Input: part model. Units: mm. Frame: model coordinates. A direction names the side the tool comes from. Coordinates: 2 decimals unless noted, no trailing zeros. Order: outer loops, then holes, each group sorted by start corner. A loop starts at its lowest first (then second) coordinate and runs counter-clockwise, first axis right, second up. Notation, with made-up numbers: M 6,19 L 29,19 A12 ccw 29,34 Z; hole C 16.5,17 d2. An arc over 180 degrees is marked long. Answer in a Markdown table with one row per item.
Autodesk Fusion 360 part; units mm, degrees
sketch "Sketch1" plane through (0, 0, 0) normal (0, 0, 1) x (1, 0, 0)
  line L0 (0, 0) -> (125, 0)
  line L1 (125, 0) -> (125, 65)
  line L2 (125, 65) -> (0, 65)
  line L3 (0, 65) -> (0, 0)
extrude "Extrude1" add sketch "Sketch1" along normal blind 30
sketch "Sketch2" plane through (0, 0, 0) normal (-1, 0, 0) x (0, -1, 0)
  line L0 (-65, 0) -> (0, 0)
  line L1 (0, 0) -> (0, 30)
  line L2 (0, 30) -> (-65, 30)
  line L3 (-65, 30) -> (-65, 0)
  line L4 (-20, 0) -> (-20, 15)
  line L5 (-20, 15) -> (-25, 15)
  line L6 (-25, 15) -> (-25, 25)
  line L7 (-25, 25) -> (-40, 25)
  line L8 (-40, 25) -> (-40, 15)
  line L9 (-40, 15) -> (-45, 15)
  line L10 (-45, 15) -> (-45, 0)
  line L11 (-45, 0) -> (-20, 0)
  dimension "d18" = 15
  dimension "d19" = 15
extrude "Extrude2" cut sketch "Sketch2" against normal blind 125 contours L0 L4 L5 L6 L7 L8 L9 L10 L11
extrude "Extrude3" cut 1 faces at (41.6667, 0, 10) along direction (0, 1, 0) blind 5
extrude "Extrude4" cut 1 faces at (83.3333, 65, 10) along direction (0, -1, 0) blind 5
extrude "Extrude5" cut 1 faces at (0, 55, 15) along direction (1, 0, 0) blind 15
sketch "Sketch3" plane through (0, 5, 0) normal (0, -1, 0) x (1, 0, 0)
  line L0 (15, 30) -> (15, 0)
  line L1 (15, 0) -> (125, 0)
  line L2 (125, 0) -> (125, 30)
  line L3 (125, 30) -> (15, 30)
  line L4 (20, 30) -> (20, 30.5)
  arc A0 (35, 50) -> (20, 30.5) centre (40.175, 30.5) ccw
  line L5 (35, 50) -> (35, 30)
extrude "Extrude6" add sketch "Sketch3" against normal blind 55 contours L3 L4 A0 L5
sketch "Sketch4" plane through (0, 0, 30) normal (0, 0, 1) x (-1, 0, 0)
  line L0 (-35, -60) -> (-35, -5)
  line L1 (-35, -5) -> (-125, -5)
  line L2 (-125, -5) -> (-125, -60)
  line L3 (-125, -60) -> (-35, -60)
sketch "Sketch5" plane through (125, 0, 0) normal (1, 0, 0) x (0, 1, 0)
  line L0 (60, 0) -> (60, 30)
  line L1 (60, 30) -> (5, 30)
  line L2 (5, 30) -> (5, 0)
  line L3 (5, 0) -> (20, 0)
  line L4 (20, 0) -> (20, 15)
  line L5 (20, 15) -> (25, 15)
  line L6 (25, 15) -> (25, 25)
  line L7 (25, 25) -> (40, 25)
  line L8 (40, 25) -> (40, 15)
  line L9 (40, 15) -> (45, 15)
  line L10 (45, 15) -> (45, 0)
  line L11 (45, 0) -> (60, 0)
  circle A0 centre (32.5, 30) radius 15
  dimension "d13" = 30
extrude "Extrude7" add sketch "Sketch5" against normal blind 15 contours L1 A0
sketch "Sketch6" plane through (0, 0, 30) normal (0, 0, 1) x (-1, 0, 0)
  line L0 (-35, -60) -> (-110, -60)
  line L1 (-110, -60) -> (-110, -5)
  line L2 (-110, -5) -> (-35, -5)
  line L3 (-35, -5) -> (-35, -60)
extrude "Extrude8" cut sketch "Sketch6" against normal blind 12.5
extrude "Extrude9" cut 2 faces at (51.6667, 15, 0) (88.3333, 50, 0) along direction (0, 0, 1) blind 5
sketch "Sketch7" plane through (110, 0, 0) normal (-1, 0, 0) x (0, -1, 0)
  arc A0 (-17.5, 30) -> (-47.5, 30) centre (-32.5, 30) ccw
  line L0 (-47.5, 30) -> (-60, 30)
  line L1 (-60, 30) -> (-60, 17.5)
  line L2 (-60, 17.5) -> (-40, 17.5)
  line L3 (-40, 17.5) -> (-40, 25)
  line L4 (-40, 25) -> (-25, 25)
  line L5 (-25, 25) -> (-25, 17.5)
  line L6 (-25, 17.5) -> (-5, 17.5)
  line L7 (-5, 17.5) -> (-5, 30)
  line L8 (-5, 30) -> (-17.5, 30)
  line L9 (-40, 17.5) -> (-41, 17.5)
  line L10 (-41, 17.5) -> (-41, 26)
  line L11 (-41, 26) -> (-24, 26)
  line L12 (-24, 26) -> (-24, 17.5)
  line L13 (-24, 17.5) -> (-25, 17.5)
  line L14 (-25, 17.5) -> (-25, 25)
  line L15 (-40, 25) -> (-40, 17.5)
  dimension "d22" = 1
  dimension "d23" = 8.5
  dimension "d24" = 17
extrude "Extrude10" add sketch "Sketch7" along normal blind 75 contours L2 L3 L4 L5 L6 L9 L10 L11 L12 L13 L14 L15
1) Material intervals for probe 1 along Y at (x, z) = (34.5, 15.5); probe 2 along Y at (x, z) = (23, 13); probe 3 along X at (y, z) = (44.5, 21.5), sorted ascending.
Resolved:
| item | result |
|---|---|
| probe 1 | y = 5 to 25, 40 to 60 |
| probe 2 | y = 5 to 20, 45 to 60 |
| probe 3 | x = 15 to 35, 110 to 125 |
2) Cut plane A-A, the plane z = 12.5. Output: boundary loops of the cut face in (x, y).
Resolved:
| item | result |
|---|---|
| outline | M 15,5 L 125,5 L 125,20 L 15,20 Z; M 15,45 L 125,45 L 125,60 L 15,60 Z |
3) Cut plane D-D, the plane z = 22. Output: boundary loops of the cut face in (x, y), and give its area (3 significant figures).
Resolved:
| item | result |
|---|---|
| outline | M 15,5 L 35,5 L 35,24 L 110,24 L 110,5 L 125,5 L 125,25 L 15,25 Z; M 15,40 L 125,40 L 125,60 L 110,60 L 110,41 L 35,41 L 35,60 L 15,60 Z |
| area | 1,550 mm2 |
4) Cut plane B-B, the plane y = 15. Output: boundary loops of the cut face in (x, z) (3 decimals), and give its area (3 significant figures).
Resolved:
| item | result |
|---|---|
| outline | M 15,5 L 125,5 L 125,30 L 110,30 L 110,17.5 L 35,17.5 L 35,50 A20.175 ccw 20,30.5 L 20,30 L 15,30 Z |
| area | 2,040 mm2 |
5) Reachability of faces 1 (the face through (69, 42, 15)), 2 (the face through (73, 33, 26)), 3 (the face through (73, 24, 22)) from +Z, -Z, +X, -X, +Y, -Y: full face, straight path, thin tool, end or side. Return the list, or none.
Resolved:
| item | result |
|---|---|
| face 1 | -Z, +X, -X |
| face 2 | +Z, +Y, -Y |
| face 3 | +Z, -Y |
6) Cut plane C-C, the plane x = 46.5. Output: boundary loops of the cut face in (y, z), and give its area (3 significant figures).
Resolved:
| item | result |
|---|---|
| outline | M 5,5 L 20,5 L 20,15 L 25,15 L 25,25 L 40,25 L 40,15 L 45,15 L 45,5 L 60,5 L 60,17.5 L 41,17.5 L 41,26 L 24,26 L 24,17.5 L 5,17.5 Z |
| area | 432 mm2 |
7) Contact query for flat-ended pins moving along their axis: pin 1 (2.5 mm diameter, centred on x = 18, y = 23.5, fed in from +Z); pin 2 (2.5 mm diameter, centred on x = 84, y = 23, fed in from -Z); pin 3 (2.5 mm diameter, centred on x = 72, z = 22, fed in from -Y); pin 4 (11 mm diameter, centred on x = 97.5, z = 21, fed in from -Y). Output: stop coordinate, or through.
Resolved:
| item | result |
|---|---|
| pin 1 | stops at z = 30 |
| pin 2 | stops at z = 15 |
| pin 3 | stops at y = 24 |
| pin 4 | stops at y = 5 |
8) Mould query, pull axis Z, two halves, no side actions, for faces 4 (the face through (117.605, 32.83, 44.996)), 5 (the face through (69, 22, 15)), 6 (the face through (35, 32, 34)). Classes: +Z half, -Z half, draft (parallel to the pull), parting line (faces both ways), or undercut.
Resolved:
| item | result |
|---|---|
| face 4 | +Z half |
| face 5 | -Z half |
| face 6 | draft |
